Could you check a few things on this model? Use its own coordinates, in mm. A direction names the side the tool comes from. Give positions to 0.01 mm unless a question says otherwise; leave off trailing zeros. Write each loop counter-clockwise with the first axis right and the second up, starting at its lowest first coordinate (ties: lowest second). Pieces come first, ordered by that corner, then holes. Notation, with made-up numbers: M 19.25,37.25 L 43.25,37.25 A17 cw 43.25,59.25 Z; hole C 85,27 d3. An arc over 180 degrees is marked long. Use one line per item in the form item = value.
from build123d import *

# Parameters (mm, degrees)
SKETCH1_R           = 2.5
SKETCH1_R_2         = 6.1
SKETCH1_R_3         = 1.55
BOSS_EXTRUDE1_DEPTH = 3
BOSS_EXTRUDE2_DEPTH = 39
BOSS_EXTRUDE3_DEPTH = 39
CUT_EXTRUDE1_DEPTH  = 3
BOSS_EXTRUDE4_DEPTH = 34
BOSS_EXTRUDE5_DEPTH = 3
CUT_EXTRUDE3_DEPTH  = 77.336426429
CUT_EXTRUDE4_START  = -10
SKETCH9_W           = 115.741675956
SKETCH9_H           = 76.731693644
SKETCH9_R           = 21
CUT_EXTRUDE4_DEPTH  = 10
SKETCH10_W          = 52.464416267
SKETCH10_H          = 51.664843315
CUT_EXTRUDE5_DEPTH  = 20


with BuildPart() as part:
    # Sketch1 → Boss-Extrude1 (new body)
    with BuildSketch(Plane.XY):
        with BuildLine():
            Line((-48.416861363, 3.650350453), (-11.959014769, 37.776226585))
            ThreePointArc((-11.959014769, 37.776226585), (0, 42.5), (11.959014769, 37.776226585))
            Line((11.959014769, 37.776226585), (48.416861363, 3.650350453))
            ThreePointArc((48.416861363, 3.650350453), (49.946989961, -0.726147591), (47.22369092, -4.478303104))
            Line((47.22369092, -4.478303104), (17.66776819, -19.154227328))
            ThreePointArc((17.66776819, -19.154227328), (16.856525691, -19.446371641), (16, -19.5455))
            Line((16, -19.5455), (-16, -19.5455))
            ThreePointArc((-16, -19.5455), (-16.856525691, -19.446371641), (-17.66776819, -19.154227328))
            Line((-17.66776819, -19.154227328), (-47.22369092, -4.478303104))
            ThreePointArc((-47.22369092, -4.478303104), (-49.946989961, -0.726147591), (-48.416861363, 3.650350453))
        make_face()
        with Locations((-25, 0)):
            Circle(SKETCH1_R, mode=Mode.SUBTRACT)
        with Locations((0, -5.5455)):
            Circle(SKETCH1_R_2, mode=Mode.SUBTRACT)
        with Locations((-7.5, 14.444881057)):
            Circle(SKETCH1_R_3, mode=Mode.SUBTRACT)
        with Locations((-15, 1.4545)):
            Circle(SKETCH1_R_3, mode=Mode.SUBTRACT)
        with Locations((-7.5, -11.535881057)):
            Circle(SKETCH1_R_3, mode=Mode.SUBTRACT)
        with Locations(Location((7.5, -11.535881057, 0), (0, 0, 180))):
            Circle(SKETCH1_R_3, mode=Mode.SUBTRACT)
        with Locations(Location((7.5, 14.444881057, 0), (0, 0, 180))):
            Circle(SKETCH1_R_3, mode=Mode.SUBTRACT)
        with Locations(Location((15, 1.4545, 0), (0, 0, 180))):
            Circle(SKETCH1_R_3, mode=Mode.SUBTRACT)
        with Locations(Location((25, 0, 0), (0, 0, 180))):
            Circle(SKETCH1_R, mode=Mode.SUBTRACT)
        with Locations((-45, 0)):
            Circle(SKETCH1_R, mode=Mode.SUBTRACT)
        with Locations(Location((45, 0, 0), (0, 0, 180))):
            Circle(SKETCH1_R, mode=Mode.SUBTRACT)
        with Locations((-16, -15.7955)):
            Circle(SKETCH1_R, mode=Mode.SUBTRACT)
        with Locations(Location((16, -15.7955, 0), (0, 0, 180))):
            Circle(SKETCH1_R, mode=Mode.SUBTRACT)
    extrude(amount=BOSS_EXTRUDE1_DEPTH)

    # Sketch2 → Boss-Extrude2 (add)
    with BuildSketch(Plane.XY.offset(3)):
        with BuildLine():
            Line((-20.75, 1.4545), (-18.75, 1.4545))
            ThreePointArc((-18.75, 1.4545), (-16.237976321, 10.8295), (-9.375, 17.692476321))
            Line((-9.375, 17.692476321), (-10.375, 19.424527129))
            ThreePointArc((-10.375, 19.424527129), (-17.970027129, 11.8295), (-20.75, 1.4545))
        make_face()
        with BuildLine():
            Line((-10.375, -16.515527129), (-9.375, -14.783476321))
            ThreePointArc((-9.375, -14.783476321), (0, -17.2955), (9.375, -14.783476321))
            Line((9.375, -14.783476321), (10.375, -16.515527129))
            ThreePointArc((10.375, -16.515527129), (0, -19.2955), (-10.375, -16.515527129))
        make_face()
        with BuildLine():
            ThreePointArc((18.75, 1.4545), (16.237976321, 10.8295), (9.375, 17.692476321))
            Line((9.375, 17.692476321), (10.375, 19.424527129))
            ThreePointArc((10.375, 19.424527129), (17.970027129, 11.8295), (20.75, 1.4545))
            Line((20.75, 1.4545), (18.75, 1.4545))
        make_face()
    extrude(amount=BOSS_EXTRUDE2_DEPTH)

    # Sketch3 → Boss-Extrude3 (add)
    with BuildSketch(Plane.XY.offset(3)):
        with BuildLine():
            Line((-17.5, 29), (-17.5, 23))
            Line((-17.5, 23), (-4, 23))
            Line((-4, 23), (-4, 20))
            Line((-4, 20), (-5.378251748, 20))
            Line((-5.378251748, 20), (-9.375, 17.692476321))
            Line((-9.375, 17.692476321), (-12.918615444, 17.692476321))
            ThreePointArc((-12.918615444, 17.692476321), (-12.502444344, 19.132335325), (-13.724553319, 20))
            Line((-13.724553319, 20), (-20.5, 20))
            Line((-20.5, 20), (-20.5, 29))
            Line((-20.5, 29), (-17.5, 29))
        make_face()
    boss_extrude3 = extrude(amount=BOSS_EXTRUDE3_DEPTH)

    # Mirror1: Boss-Extrude3 across plane
    add(boss_extrude3.mirror(Plane(origin=(0, 0, 0), x_dir=(0, 0, 1), z_dir=(1, 0, 0))))

    # Sketch4 → Cut-Extrude1 (cut)
    with BuildSketch(Plane(origin=(0, 23, 0), x_dir=(1, 0, 0), z_dir=(0, 1, 0))):
        with BuildLine():
            Line((-14.224553319, -17.5), (-14.224553319, -27.5))
            ThreePointArc((-14.224553319, -27.5), (-15.724553319, -29), (-17.224553319, -27.5))
            Line((-17.224553319, -27.5), (-17.224553319, -17.5))
            ThreePointArc((-17.224553319, -17.5), (-15.724553319, -16), (-14.224553319, -17.5))
        make_face()
        with BuildLine():
            Line((14.224553319, -17.5), (14.224553319, -27.5))
            ThreePointArc((14.224553319, -27.5), (15.724553319, -29), (17.224553319, -27.5))
            Line((17.224553319, -27.5), (17.224553319, -17.5))
            ThreePointArc((17.224553319, -17.5), (15.724553319, -16), (14.224553319, -17.5))
        make_face()
    extrude(amount=-CUT_EXTRUDE1_DEPTH, mode=Mode.SUBTRACT)

    # Sketch5 → Boss-Extrude4 (add)
    with BuildSketch(Plane.XY.offset(3)):
        Polygon((-43.784396435, 23.346849864), (-43.784396435, 6.040412882), (-29.176551712, -7.739510205), (-18.086117895, -7.739510205), (-18.086117895, -4.739510205), (-27.984845454, -4.739510205), (-40.784396435, 7.334606915), (-40.784396435, 23.346849864), align=None)
    boss_extrude4 = extrude(amount=BOSS_EXTRUDE4_DEPTH)

    # Mirror2: Boss-Extrude4 across plane
    add(boss_extrude4.mirror(Plane(origin=(0, 0, 0), x_dir=(0, 0, 1), z_dir=(1, 0, 0))))

    # Sketch6 → Boss-Extrude5 (add)
    with BuildSketch(Plane(origin=(0, 0, 3), x_dir=(-1, 0, 0), z_dir=(0, 0, -1))):
        Polygon((40.784396435, 23.346849864), (40.784396435, 10.794616422), (43.784396435, 7.986506839), (43.784396435, 23.346849864), align=None)
        Polygon((-43.784396435, 23.346849864), (-43.784396435, 7.986506839), (-40.784396435, 10.794616422), (-40.784396435, 23.346849864), align=None)
    extrude(amount=BOSS_EXTRUDE5_DEPTH)

    # Sketch8 → Cut-Extrude3 (cut, through all)
    with BuildSketch(Plane.XY.offset(3)):
        with BuildLine():
            Line((50.685566108, 53.585257373), (-51.78645156, 53.585257373))
            Line((-51.78645156, 53.585257373), (-51.78645156, -24.701187201))
            Line((-51.78645156, -24.701187201), (50.685566108, -24.701187201))
            Line((50.685566108, -24.701187201), (50.685566108, -10.970768248))
            Line((50.685566108, -10.970768248), (16.929639954, -10.970768248))
            ThreePointArc((16.929639954, -10.970768248), (0, -19.5455), (-16.929639954, -10.970768248))
            Line((-16.929639954, -10.970768248), (-24.865040571, -10.970768248))
            Line((-24.865040571, -10.970768248), (-24.865040571, -1.968887806))
            Line((-24.865040571, -1.968887806), (-20.719083376, -1.968887806))
            ThreePointArc((-20.719083376, -1.968887806), (-1.717447104, 22.384153018), (21, 1.4545))
            ThreePointArc((21, 1.4545), (20.929653018, -0.262947104), (20.719083376, -1.968887806))
            Line((20.719083376, -1.968887806), (50.685566108, -1.968887806))
            Line((50.685566108, -1.968887806), (50.685566108, 53.585257373))
        make_face()
        with BuildLine():
            ThreePointArc((16.929639954, -10.970768248), (19.354974941, -6.693195689), (20.719083376, -1.968887806))
            Line((20.719083376, -1.968887806), (-20.719083376, -1.968887806))
            ThreePointArc((-20.719083376, -1.968887806), (-19.354974941, -6.693195689), (-16.929639954, -10.970768248))
            Line((-16.929639954, -10.970768248), (16.929639954, -10.970768248))
        make_face()
        with BuildLine():
            ThreePointArc((-16.929639954, -10.970768248), (-19.354974941, -6.693195689), (-20.719083376, -1.968887806))
            Line((-20.719083376, -1.968887806), (-24.865040571, -1.968887806))
            Line((-24.865040571, -1.968887806), (-24.865040571, -10.970768248))
            Line((-24.865040571, -10.970768248), (-16.929639954, -10.970768248))
        make_face()
        with BuildLine():
            Line((50.685566108, -10.970768248), (50.685566108, -1.968887806))
            Line((50.685566108, -1.968887806), (20.719083376, -1.968887806))
            ThreePointArc((20.719083376, -1.968887806), (19.354974941, -6.693195689), (16.929639954, -10.970768248))
            Line((16.929639954, -10.970768248), (50.685566108, -10.970768248))
        make_face()
    extrude(amount=CUT_EXTRUDE3_DEPTH, mode=Mode.SUBTRACT)

    # Sketch9 → Cut-Extrude4 (cut)
    with BuildSketch(Plane.XY.offset(3).offset(CUT_EXTRUDE4_START)):
        with Locations((-2.250274658, 10.895525105)):
            Rectangle(SKETCH9_W, SKETCH9_H)
        with Locations(Location((0, 1.4545, 0), (0, 0, 126.468628992))):
            Circle(SKETCH9_R, mode=Mode.SUBTRACT)
    extrude(amount=CUT_EXTRUDE4_DEPTH, mode=Mode.SUBTRACT)

    # Sketch10 → Cut-Extrude5 (cut)
    with BuildSketch(Plane.XY.offset(42)):
        with Locations((-1.737703473, -0.030968104)):
            Rectangle(SKETCH10_W, SKETCH10_H)
    extrude(amount=-CUT_EXTRUDE5_DEPTH, mode=Mode.SUBTRACT)


solid = part.part
1) I want a section at C-C, the plane y = 2. Please give me the cut outline in (x, z).
Checked values:
outline = M -20.99,0 L -16.45,0 L -16.45,3 L -18.74,3 L -18.74,22 L -20.74,22 L -20.74,3 L -20.99,3 Z; M -13.55,0 L 13.55,0 L 13.55,3 L -13.55,3 Z; M 16.45,0 L 20.99,0 L 20.99,3 L 20.74,3 L 20.74,22 L 18.74,22 L 18.74,3 L 16.45,3 Z
2) If I drill on L1, parallel to Y at x = 0, z = 1.6; L2, parallel to Y at x = -7.5, z = 1.15; L3, parallel to Z at x = 13, y = 1, over which ranges is the centre line in solid material (lowest first)?
Checked values:
L1 = -19.55 to -11.65, 0.55 to 22.45
L2 = -18.16 to -13.09, -9.99 to 12.89, 15.99 to 21.07
L3 = 0 to 3
3) For pin 1 Ø0.6 at (x, z) = (20, 15) entering from -Y; pin 2 Ø5 at (y, z) = (16, 14) entering from +X; pin 3 Ø4 at (x, y) = (7.5, -11.54) entering from +Z, each with a flat end and sliding along its axis, tell me the tip position at first contact or that it passes through.
Checked values:
pin_1 = 1.45
pin_2 = 16.9
pin_3 = 3
4) I want a section at A-A, the plane z = 20.5. Count the separate pieces of the cut face and the enclosed holes in it, plus the area to 3 significant figures.
Checked values:
separate_pieces = 3
enclosed_holes = 0
area = 151 mm2
5) I want a section at B-B, the plane x = 0. Please give me the cut outline in (y, z).
Checked values:
outline = M -19.55,0 L -11.65,0 L -11.65,3 L -17.3,3 L -17.3,22 L -19.3,22 L -19.3,3 L -19.55,3 Z; M 0.55,0 L 22.45,0 L 22.45,3 L 0.55,3 Z
6) For faces 1 (the cylindrical face through (18.63, 10.59, 12.37)), 2 (the cylindrical face through (0.152, -19.295, 12.367)), 3 (the flat face through (7.35, 18.86, 12.37)), 4 (the flat face through (9.87, -15.64, 12.37)), 5 (the flat face through (-4, 21, 12)), which set-ups out of +Z, -Z, +X, -X, +Y, -Y let a thin tool reach every point of the face, with its end or its side?
Checked values:
face_1 = +Z, +X, +Y
face_2 = +Z, -Y
face_3 = +Z
face_4 = +Z, +X
face_5 = +Z, +Y
7) I want a section at D-D, the plane x = 7.5. Please give me the cut outline in (y, z) (3 decimals).
Checked values:
outline = M -18.161,0 L -13.086,0 L -13.086,3 L -15.73,3 L -15.73,22 L -17.893,22 L -17.893,3 L -18.161,3 Z; M -9.986,0 L 12.895,0 L 12.895,3 L -9.986,3 Z; M 15.995,0 L 21.07,0 L 21.07,22 L 18.775,22 L 18.775,3 L 15.995,3 Z
8) Thinking about a two-plate mould opening in Y: for faces 6 (the flat face through (-9.88, -15.66, 12.37)), 7 (the flat face through (15, 14, 22)), 8 (the flat face through (-20, 1.454, 12)), which applies, released by +Y, released by -Y, zero draft, split by the parting line, or undercut?
Checked values:
face_6 = undercut
face_7 = zero draft
face_8 = released by -Y
